```python
from build123d import *

# Parameters (mm, degrees)
F0_W      = 97
F0_H      = 77
F1_DEPTH  = 2
F2_W      = 89.8
F2_H      = 69.8
F3_DEPTH  = 1
F4_W      = 4
F4_H      = 10
F5_DEPTH  = 10
F6_R      = 4.99999
F7_R      = 1.4
F8_DEPTH  = 93.401
F10_DEPTH = 2
F11_W     = 97
F11_H     = 77
F11_W_2   = 88.8
F11_H_2   = 68.8
F12_DEPTH = 11.001
F13_SIZE  = 0.5
F14_SIZE  = 0.4


# Not quite as in the source:
# - a fillet or chamfer is up to 0.001 mm smaller than in the source, because OpenCascade refuses the exact size


with BuildPart() as f1:
    # F0 (on Top) → F1 (new body)
    with BuildSketch(Plane.XY):
        Rectangle(F0_W, F0_H)
    extrude(amount=F1_DEPTH)

    # F2 (on face) → F3 (join)
    with BuildSketch(Plane.XY.offset(2)):
        Rectangle(F2_W, F2_H)
    extrude(amount=F3_DEPTH)

    # F4 (on face) → F5 (join)
    with BuildSketch(Plane.XY.offset(3)):
        with Locations((-42.9, 29.9)):
            Rectangle(F4_W, F4_H)
        with Locations((42.9, 29.9)):
            Rectangle(F4_W, F4_H)
        with Locations((-42.9, -29.9)):
            Rectangle(F4_W, F4_H)
        with Locations((42.9, -29.9)):
            Rectangle(F4_W, F4_H)
    extrude(amount=F5_DEPTH)

    # F6 (radius 5 in the source; OpenCascade refuses exactly that, so slightly less here)
    f6_edges = [f1.edges().sort_by_distance(p)[0] for p in [
        (42.9, 34.9, 13),
        (42.9, 24.9, 13),
        (42.9, -24.9, 13),
        (42.9, -34.9, 13),
        (-42.9, -24.9, 13),
        (-42.9, -34.9, 13),
        (-42.9, 34.9, 13),
        (-42.9, 24.9, 13),
    ]]
    fillet(f6_edges, radius=F6_R)

    # F7 (on face) → F8 (cut, through all)
    with BuildSketch(Plane(origin=(-44.9, 0, 0), x_dir=(0, -1, 0), z_dir=(-1, 0, 0))):
        with Locations((-29.9, 8)):
            Circle(F7_R)
        with Locations((29.9, 8)):
            Circle(F7_R)
    extrude(amount=-F8_DEPTH, mode=Mode.SUBTRACT)

    # F9 (on face) → F10 (cut)
    with BuildSketch(Plane.XY.offset(3)):
        Polygon((-42.9, -22.9), (-38.9, -22.9), (-38.9, -32.9), (38.9, -32.9), (38.9, -22.9), (42.9, -22.9), (42.9, 22.9), (38.9, 22.9), (38.9, 32.9), (-38.9, 32.9), (-38.9, 22.9), (-42.9, 22.9), align=None)
    extrude(amount=-F10_DEPTH, mode=Mode.SUBTRACT)

    # F11 (on face) → F12 (cut, through all)
    with BuildSketch(Plane.XY.offset(2)):
        Rectangle(F11_W, F11_H)
        Rectangle(F11_W_2, F11_H_2, mode=Mode.SUBTRACT)
    extrude(amount=F12_DEPTH, mode=Mode.SUBTRACT)

    # F13
    f13_edges = [f1.edges().sort_by_distance(p)[0] for p in [
        (44.4, 0, 3),
        (0, -34.4, 3),
        (-44.4, 0, 3),
        (0, 34.4, 3),
    ]]
    chamfer(f13_edges, length=F13_SIZE)

    # F14
    f14_edges = [f1.edges().sort_by_distance(p)[0] for p in [
        (-48.5, 0, 2),
        (0, 38.5, 2),
        (48.5, 0, 2),
        (0, -38.5, 2),
    ]]
    chamfer(f14_edges, length=F14_SIZE)


solid = f1.part
```
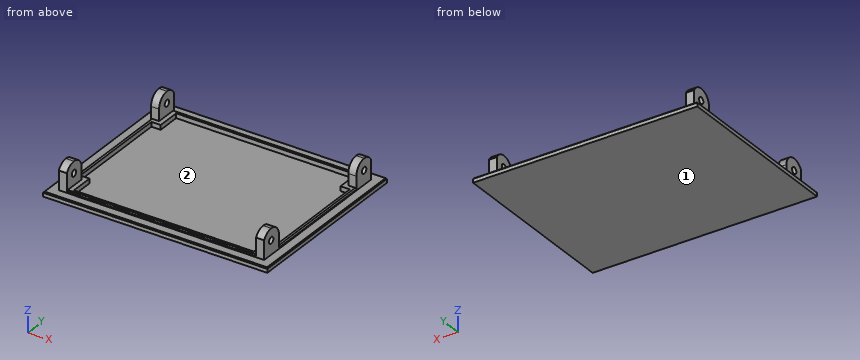
Read the model definition and answer for the solid it produces. Units are mm, in the model's axes. Face numbers are marked on the shaded views. Round coordinates to 2 decimals unless told otherwise and drop trailing zeros. Write each loop counter-clockwise with the first axis right and the second up, starting at its lowest first coordinate (ties: lowest second). Pieces come first, ordered by that corner, then holes. Notation, with made-up numbers: M 70,14.25 L 96,14.25 A11 cw 96,23.25 Z; hole C 86.5,33 d2. An arc over 180 degrees is marked long. One line per item, written item: value.
Q1. Find section B-B on x = -2. Write down the section's boundary in (y, z).
Data:
outline: M -38.5,0 L 38.5,0 L 38.5,1.6 L 38.1,2 L 34.4,2 L 34.4,2.5 L 33.9,3 L 32.9,3 L 32.9,1 L -32.9,1 L -32.9,3 L -33.9,3 L -34.4,2.5 L -34.4,2 L -38.1,2 L -38.5,1.6 Z
Q2. Find section C-C on y = -18.5. Write down the section's boundary in (x, z), plus the area to 3 significant figures.
Data:
outline: M -48.5,0 L 48.5,0 L 48.5,1.6 L 48.1,2 L 44.4,2 L 44.4,2.5 L 43.9,3 L 42.9,3 L 42.9,1 L -42.9,1 L -42.9,3 L -43.9,3 L -44.4,2.5 L -44.4,2 L -48.1,2 L -48.5,1.6 Z
area: 111 mm2
Q3. Find section D-D on z = 11.5. Write down the section's boundary in (x, y), plus the area to 4 significant figures.
Data:
outline: M -44.4,-33.47 L -40.9,-33.47 L -40.9,-26.33 L -44.4,-26.33 Z; M -44.4,26.33 L -40.9,26.33 L -40.9,33.47 L -44.4,33.47 Z; M 40.9,-33.47 L 44.4,-33.47 L 44.4,-26.33 L 40.9,-26.33 Z; M 40.9,26.33 L 44.4,26.33 L 44.4,33.47 L 40.9,33.47 Z
area: 100.0 mm2
Q4. Straight lines are drawn through the part: line 1 (Z direction, x = -43.4, y = -29.9); line 2 (X direction, y = -32, z = 4); line 3 (Y direction, x = -12, z = 1.5). For each, find the intervals that lie inside material, in ascending order. Write a range as [from, to].
Data:
line 1: [0, 6.6], [9.4, 13]
line 2: [-44.4, -40.9], [40.9, 44.4]
line 3: [-38.5, -32.9], [32.9, 38.5]
Q5. Find section A-A on z = 4.25. Write down the section's boundary in (x, y).
Data:
outline: M -44.4,-34.4 L -40.9,-34.4 L -40.9,-24.9 L -44.4,-24.9 Z; M -44.4,24.9 L -40.9,24.9 L -40.9,34.4 L -44.4,34.4 Z; M 40.9,-34.4 L 44.4,-34.4 L 44.4,-24.9 L 40.9,-24.9 Z; M 40.9,24.9 L 44.4,24.9 L 44.4,34.4 L 40.9,34.4 Z
Q6. For a pull along Y with two mould halves and no side action, classify the marked faces 1 and 2 as +Y half, -Y half, draft (parallel to the pull), parting line (faces both ways), or undercut.
Data:
face 1: draft
face 2: undercut
Q7. Flat-ended cylindrical pins translate along their axes: pin 1 Ø20.5 at (x, y) = (12.5, 11.5) entering from +Z; pin 2 Ø0.6 at (y, z) = (5, 2) entering from -X; pin 3 Ø7.5 at (y, z) = (30.5, 7) entering from +X. Find the tip coordinate at first contact, or state that the pin passes through.
Data:
pin 1: z = 1
pin 2: x = -48.4
pin 3: x = 44.4
